Geometry check sheet. Reference: the model listing, model coordinates, mm. A direction names the side the tool comes from. Give positions to 0.01 mm unless a question says otherwise; leave off trailing zeros. Write each loop counter-clockwise with the first axis right and the second up, starting at its lowest first coordinate (ties: lowest second). Pieces come first, ordered by that corner, then holes.
(1) Cross-section at C-C (y = 57.75). Record the boundary of the cut face in (x, z), and give its area (3 significant figures).
(2) Cross-section at B-B (x = -171). Record the boundary of the cut face in (y, z), and give its area (3 significant figures).
(3) Mould release check, pull along Z, two halves, no side actions. Record for faces 4 (the flat face through (-170, 47, 104)), 5 (the flat face through (-163.5, 56.6, 137)), 6 (the cylindrical face through (-169.395, 51.33, 84.883)): +Z half, -Z half, draft (parallel to the pull), parting line (faces both ways), or undercut.
(4) Thickness scan on line 1 along Z through (x, y) = (-171, 56); line 2 along Y through (x, z) = (-173.25, 86.5); line 3 along Z through (x, y) = (-171.5, 48.25). Record the ranges inside material, lowest first.
(5) Tool access check on faces 1 (the flat face through (-171, 55, 138.5)), 2 (the flat face through (-171, 62, 123)), 3 (the flat face through (-171, 62, 136)). Record the directions out of +Z, -Z, +X, -X, +Y, -Y that give a thin tool (end or side, any length) a straight path to the whole face; none if there is none.
(6) Cross-section at A-A (y = 52). Record the boundary of the cut face in (x, z), and give its area (3 significant figures).
(7) Depth check by flat-ended pin: P1, Ø0.6, axis at x = -170.5, z = 108.5, coming from the -Y side. Enter the tip coordinate at first touch or a pass-through.
(8) Cross-section at D-D (z = 108.75). Record the boundary of the cut face in (x, y).
```python
from build123d import *

# Parameters (mm, degrees)
CROQUIS1_W              = 19
CROQUIS1_H              = 56
SALIENTE_EXTRUIR1_DEPTH = 15
CHAFL_N1_SIZE           = 3
CROQUIS2_W              = 12.5
CROQUIS2_H              = 24
CORTAR_EXTRUIR1_DEPTH   = 15
CROQUIS3_R              = 1
CORTAR_EXTRUIR2_DEPTH   = 15
CROQUIS8_R              = 1
CORTAR_EXTRUIR3_DEPTH   = 15
CROQUIS9_R              = 1.75
CORTAR_EXTRUIR4_DEPTH   = 16
CORTAR_EXTRUIR5_REACH   = 17
CROQUIS10_R             = 1.75
CROQUIS11_R             = 1.75
CORTAR_EXTRUIR6_DEPTH   = 20
CROQUIS12_R             = 1.75
CORTAR_EXTRUIR7_DEPTH   = 2


with BuildPart() as part:
    # Croquis1 → Saliente-Extruir1 (new body)
    with BuildSketch(Plane(origin=(-177, 0, 0), x_dir=(0, -1, 0), z_dir=(-1, 0, 0))):
        with Locations((-56.5, 110.5)):
            Rectangle(CROQUIS1_W, CROQUIS1_H)
    extrude(amount=-SALIENTE_EXTRUIR1_DEPTH)

    # Chaflán1
    chafl_n1_edges = [part.edges().sort_by_distance(p)[0] for p in [
        (-162, 56.5, 138.5),
        (-169.5, 66, 138.5),
    ]]
    chamfer(chafl_n1_edges, length=CHAFL_N1_SIZE)

    # Croquis2 → Cortar-Extruir1 (cut)
    with BuildSketch(Plane.XZ.offset(-47)):
        with Locations((-170.75, 122.5)):
            Rectangle(CROQUIS2_W, CROQUIS2_H)
    extrude(amount=-CORTAR_EXTRUIR1_DEPTH, mode=Mode.SUBTRACT)

    # Croquis3 → Cortar-Extruir2 (cut)
    with BuildSketch(Plane.XZ.offset(-47)):
        with Locations((-171, 136.25)):
            Circle(CROQUIS3_R)
    extrude(amount=-CORTAR_EXTRUIR2_DEPTH, mode=Mode.SUBTRACT)

    # Croquis8 → Cortar-Extruir3 (cut)
    with BuildSketch(Plane(origin=(0, 47, 0), x_dir=(-1, 0, 0), z_dir=(0, -1, 0))):
        with Locations((171, -108.75)):
            Circle(CROQUIS8_R)
    extrude(amount=-CORTAR_EXTRUIR3_DEPTH, mode=Mode.SUBTRACT)

    # Croquis9 → Cortar-Extruir4 (cut, through all)
    with BuildSketch(Plane(origin=(-162, 0, 0), x_dir=(0, 0, -1), z_dir=(1, 0, 0))):
        with Locations((-86.5, 52)):
            Circle(CROQUIS9_R)
    extrude(amount=-CORTAR_EXTRUIR4_DEPTH, mode=Mode.SUBTRACT)

    # Croquis10 → Cortar-Extruir5 (cut, up to next)
    with BuildSketch(Plane(origin=(-162, 0, 0), x_dir=(0, 0, -1), z_dir=(1, 0, 0)), mode=Mode.PRIVATE) as cortar_extruir5_sk1:
        with Locations((-86.5, 62)):
            Circle(CROQUIS10_R)
    cortar_extruir5_tool1 = extrude(cortar_extruir5_sk1.sketch, amount=-CORTAR_EXTRUIR5_REACH, mode=Mode.PRIVATE) & part.part
    add(cortar_extruir5_tool1.solids().sort_by_distance((-162, 62, 86.5))[0], mode=Mode.SUBTRACT)

    # Croquis11 → Cortar-Extruir6 (cut, through all)
    with BuildSketch(Plane(origin=(0, 66, 0), x_dir=(-1, 0, 0), z_dir=(0, 1, 0))):
        with Locations((171, 128.35)):
            Circle(CROQUIS11_R)
    extrude(amount=-CORTAR_EXTRUIR6_DEPTH, mode=Mode.SUBTRACT)

    # Croquis12 → Cortar-Extruir7 (cut)
    with BuildSketch(Plane.XZ.offset(-62)):
        Polygon((-172.65, 125.492116168), (-169.35, 125.492116168), (-167.7, 128.35), (-169.35, 131.207883832), (-172.65, 131.207883832), (-174.3, 128.35), align=None)
        with Locations((-171, 128.35)):
            Circle(CROQUIS12_R, mode=Mode.SUBTRACT)
    extrude(amount=-CORTAR_EXTRUIR7_DEPTH, mode=Mode.SUBTRACT)


solid = part.part
```
Reply:
1. outline: (-177, 82.5) - (-162, 82.5) - (-162, 135.5) - (-165, 138.5) - (-177, 138.5) - (-177, 134.5) - (-164.5, 134.5) - (-164.5, 110.5) - (-177, 110.5) - close; hole circle Ø2 at (-171, 108.75); hole circle Ø2 at (-171, 136.25)
1. area: 529 mm2
2. outline: (47, 82.5) - (66, 82.5) - (66, 126.6) - (64, 126.6) - (64, 125.49) - (62, 125.49) - (62, 110.5) - (47, 110.5) - (47, 109.75) - (62, 109.75) - (62, 107.75) - (47, 107.75) - close; (47, 134.5) - (62, 134.5) - (62, 131.21) - (64, 131.21) - (64, 130.1) - (66, 130.1) - (66, 135.5) - (63, 138.5) - (47, 138.5) - (47, 137.25) - (62, 137.25) - (62, 135.25) - (47, 135.25) - close; hole circle Ø3.5 at (52, 86.5); hole circle Ø3.5 at (62, 86.5)
2. area: 602 mm2
3. face 4: draft
3. face 5: +Z half
3. face 6: undercut
4. line 1: z = 82.5 to 107.75, 109.75 to 110.5, 134.5 to 135.25, 137.25 to 138.5
4. line 2: y = 47 to 50.25, 53.75 to 60.25, 63.75 to 66
4. line 3: z = 82.5 to 107.88, 109.62 to 110.5, 134.5 to 135.38, 137.12 to 138.5
5. face 1: +Z, +X, -X, +Y, -Y
5. face 2: -X, -Y
5. face 3: -Y
6. outline: (-177, 82.5) - (-162, 82.5) - (-162, 84.75) - (-177, 84.75) - close; (-177, 88.25) - (-162, 88.25) - (-162, 135.5) - (-165, 138.5) - (-177, 138.5) - (-177, 134.5) - (-164.5, 134.5) - (-164.5, 110.5) - (-177, 110.5) - close; hole circle Ø2 at (-171, 108.75); hole circle Ø2 at (-171, 136.25)
6. area: 477 mm2
7. P1: stops at y = 62
8. outline: (-177, 47) - (-172, 47) - (-172, 62) - (-170, 62) - (-170, 47) - (-162, 47) - (-162, 66) - (-177, 66) - close
